from build123d import *

# Parameters (mm, degrees)
BOSS_EXTRUDE1_DEPTH = 7.5


with BuildPart() as part:
    # Sketch1 → Boss-Extrude1 (new body)
    with BuildSketch(Plane(origin=(0, 0, 0), x_dir=(1, 0, 0), z_dir=(0, 1, 0))):
        with BuildLine():
            Line((0, 0), (-150, 0))
            Line((-150, 0), (-150, -55))
            Line((-150, -55), (-175, -55))
            ThreePointArc((-175, -55), (-225, -105), (-175, -155))
            Line((-175, -155), (-150, -155))
            Line((-150, -155), (-150, -210))
            Line((-150, -210), (0, -210))
            Line((0, -210), (0, 0))
        make_face()
        with BuildLine():
            Line((-175, -75), (-175, -135))
            ThreePointArc((-175, -135), (-205, -105), (-175, -75))
        make_face(mode=Mode.SUBTRACT)
    extrude(amount=BOSS_EXTRUDE1_DEPTH)


solid = part.part
The model under review builds one solid part; all positions refer to its coordinate system, in mm. A direction names the side the tool comes from. Round coordinates to 2 decimals unless told otherwise and drop trailing zeros. Order: outer loops, then holes, each group sorted by start corner. A loop starts at its lowest first (then second) coordinate and runs counter-clockwise, first axis right, second up. Notation, with made-up numbers: (44.5, -19) -> (90.5, -19) arc R25 cw to (90.5, 20) -> close; hole circle Ø3 at (13, 30). An arc over 180 degrees is marked (long way). Use CSV: the item, a comma, the result in double quotes. Start each with the question number.
(1) Consider section B-B on z = 115. Write out the cut boundary in (x, y).
(2) Wall thickness on probe 1 along X at (y, z) = (4.25, 9); probe 2 along X at (y, z) = (4.25, 102); probe 3 along X at (y, z) = (7.25, 65): over which ranges is each line inside the solid? List them lowest first. Write a range as from..to.
(3) Mouldability with a two-part tool opening along Z and no side actions: class faces 4 (the face through (-175, 4, 105)), 5 (the face through (-224.988, 3.698, 103.901)), 6 (the face through (-89, 7.5, 104)) as pulls with the +Z half, pulls with the -Z half, needs draft (parallel to the pull), parting line crosses it, or undercut.
(4) Consider section D-D on z = 88. Write out the cut boundary in (x, y), and give its area (3 significant figures).
(5) Consider section C-C on z = 186. Write out the cut boundary in (x, y).
(6) Consider section A-A on y = 6.25. Write out the cut boundary in (x, z), and give its area (3 significant figures).
(7) Insertion check: pin 1 (4 mm diameter, centred on y = 4.5, z = 103, fed in from -X); pin 2 (3 mm diameter, centred on y = 5, z = 60.5, fed in from -X); pin 3 (2 mm diameter, centred on y = 2.5, z = 15.5, fed in from -X). Each pin has a flat end and moves straight along its axis. Give the tip position at first contact, or say it passes through.
(8) Tool access review of faces 1 (the face through (-162, 4, 55)), 2 (the face through (-204.993, 3.698, 105.66)), 3 (the face through (-163, 4, 155)): name each direction out of +Z, -Z, +X, -X, +Y, -Y from which nothing blocks a thin tool from reaching the whole face with its end or side.
Responses:
1,outline,"(-223.99, 0) -> (-203.28, 0) -> (-203.28, 7.5) -> (-223.99, 7.5) -> close; (-175, 0) -> (0, 0) -> (0, 7.5) -> (-175, 7.5) -> close"
2,probe 1,"-150..0"
2,probe 2,"-224.91..-204.85, -175..0"
2,probe 3,"-205..0"
3,face 4,"undercut"
3,face 5,"parting line crosses it"
3,face 6,"needs draft"
4,outline,"(-222.02, 0) -> (-199.72, 0) -> (-199.72, 7.5) -> (-222.02, 7.5) -> close; (-175, 0) -> (0, 0) -> (0, 7.5) -> (-175, 7.5) -> close"
4,area,"1,480 mm²"
5,outline,"(-150, 0) -> (0, 0) -> (0, 7.5) -> (-150, 7.5) -> close"
6,outline,"(-175, 55) -> (-150, 55) -> (-150, 0) -> (0, 0) -> (0, 210) -> (-150, 210) -> (-150, 155) -> (-175, 155) arc R50 ccw to start; hole (-175, 75) -> (-175, 135) arc R30 ccw to start"
6,area,"36,500 mm²"
7,pin 1,"x = -225"
7,pin 2,"x = -200.51"
7,pin 3,"x = -150"
8,face 1,"-Z, -X, +Y, -Y"
8,face 2,"+Y, -Y"
8,face 3,"+Z, -X, +Y, -Y"
